Autodesk Inventor part; units mm, degrees
ref_plane "YZ Plane" through (0, 0, 0) normal (1, 0, 0) x (0, 1, 0)
ref_plane "XZ Plane" through (0, 0, 0) normal (0, 1, 0) x (-1, 0, 0)
ref_plane "XY Plane" through (0, 0, 0) normal (0, 0, 1) x (1, 0, 0)
sketch "Sketch1" plane through (0, 0, 0) normal (1, 0, 0) x (0, 1, 0)
  line L0 (0, 0) -> (0, 30)
  line L1 (-11.5, 30) -> (-11.5, 2.5)
  line L2 (-11.5, 2.5) -> (-13, 2.5)
  line L3 (-13, 2.5) -> (-13, 0)
  line L4 (-13, 0) -> (-20, 0)
  line L5 (-20, 0) -> (-20, 3)
  line L6 (-20, 3) -> (-13.5, 4.7417)
  line L7 (-13.5, 4.7417) -> (-13.5, 30)
  line L8 (-13.5, 30) -> (-11.5, 30)
  dimension "d0" = 30
  dimension "d1" = 27
  dimension "d2" = 26
  dimension "d3" = 2.5
  dimension "d4" = 23
  dimension "d5" = 15
  dimension "d6" = 3
  dimension "d7" = 40
revolve "Revolution1" add sketch "Sketch1" angle 360 about axis through (0, 0, 0) along (0, 0, 1)
fillet "Fillet1" radius 1 2 edges at (0, 20, 3) (0, 13.5, 4.7417)
chamfer "Chamfer1" distance 0.2 angle 45 4 edges at (0, 20, 0) (0, 13, 0) (0, 11.5, 2.5) (0, 13, 2.5)
properties part number "nw-25-welded-30" material "Stainless Steel"
Read the model definition and answer for the solid it produces. Units are mm, in the model's axes. A direction names the side the tool comes from. Round coordinates to 2 decimals unless told otherwise and drop trailing zeros. Order: outer loops, then holes, each group sorted by start corner. A loop starts at its lowest first (then second) coordinate and runs counter-clockwise, first axis right, second up.
1) Flat-ended cylindrical pins translate along their axes: pin 1 (2 mm diameter, centred on x = 8.5, z = 26.5, fed in from -Y) (3 decimals); pin 2 (12 mm diameter, centred on x = 2.5, y = 13.5, fed in from -Z); pin 3 (1.5 mm diameter, centred on x = -5.5, z = 6, fed in from -Y); pin 4 (1 mm diameter, centred on y = -2, z = 19.5, fed in from -X). Find the tip coordinate at first contact, or state that the pin passes through.
2) Straight lines are drawn through the part: L1, parallel to X at y = 0, z = 1.65; L2, parallel to Y at x = 0.5, z = 5; L3, parallel to X at y = 1.5, z = 3. For each, find the intervals that lie inside material, in ascending order.
3) The mould has two halves that part along Y. Classify faces 4 (the face through (-4, -13, 0)), 5 (the face through (12.91, -6.72, 4.46)), 6 (the face through (-11.4, 1.5, 16.2)), 7 (the face through (7.91, 10.316, 1.235)): released by +Y, released by -Y, zero draft, split by the parting line, or undercut.
4) For faces 1 (the face through (-13.18, 2.93, 17.93)), 2 (the face through (-3.7, -11.3, 2.5)), 3 (the face through (6, -10, 30)), determine the directions among +Z, -Z, +X, -X, +Y, -Y from which every point of the face is accessible in a straight line to the end or side of a thin tool.
5) The part is cut by section A-A on z = 22. Write down the section's boundary in (x, y), plus the area to 3 significant figures.
Resolved:
1. pin 1: stops at y = -11.225
1. pin 2: stops at z = 0
1. pin 3: stops at y = -12.64
1. pin 4: stops at x = -13.42
2. L1: x = -20 to -13, 13 to 20
2. L2: y = -13.63 to -11.49, 11.49 to 13.63
2. L3: x = -19.58 to -11.4, 11.4 to 19.58
3. face 4: zero draft
3. face 5: split by the parting line
3. face 6: undercut
3. face 7: undercut
4. face 1: +Z
4. face 2: -Z
4. face 3: +Z, +X, -X, +Y, -Y
5. outline: circle Ø27 at (0, 0); hole circle Ø23 at (0, 0)
5. area: 157 mm2
